Here's how the part is built. I have some questions about the finished solid (model axes, mm). A direction names the side the tool comes from. Coordinates: 2 decimals unless noted, no trailing zeros. Write each loop counter-clockwise with the first axis right and the second up, starting at its lowest first coordinate (ties: lowest second). Pieces come first, ordered by that corner, then holes.
```python
from build123d import *

# Parameters (mm, degrees)
F1_DEPTH = 87.5
F3_DEPTH = 100
F4_R     = 6.25
F5_DEPTH = 60.001
F6_R     = 3
F7_DEPTH = 120.001


with BuildPart() as f1:
    # F0 (on Top) → F1 (new body, symmetric)
    with BuildSketch(Plane.XY):
        with BuildLine():
            Line((20, 30), (-20, 30))
            ThreePointArc((-20, 30), (-27.071068, 27.071068), (-30, 20))
            Line((-30, 20), (-30, -20))
            ThreePointArc((-30, -20), (-27.071068, -27.071068), (-20, -30))
            Line((-20, -30), (20, -30))
            ThreePointArc((20, -30), (27.071068, -27.071068), (30, -20))
            Line((30, -20), (30, 20))
            ThreePointArc((30, 20), (27.071068, 27.071068), (20, 30))
        make_face()
        with BuildLine():
            ThreePointArc((-25, 20), (-23.535534, 23.535534), (-20, 25))
            Line((-20, 25), (20, 25))
            ThreePointArc((20, 25), (23.535534, 23.535534), (25, 20))
            Line((25, 20), (25, -20))
            ThreePointArc((25, -20), (23.535534, -23.535534), (20, -25))
            Line((20, -25), (-20, -25))
            ThreePointArc((-20, -25), (-23.535534, -23.535534), (-25, -20))
            Line((-25, -20), (-25, 20))
        make_face(mode=Mode.SUBTRACT)
    extrude(amount=F1_DEPTH, both=True)

    # F2 (on Front) → F3 (join, symmetric)
    with BuildSketch(Plane.XZ):
        with BuildLine():
            Line((-40, -27.5), (-80, -27.5))
            ThreePointArc((-80, -27.5), (-87.071068, -30.428932), (-90, -37.5))
            Line((-90, -37.5), (-90, -77.5))
            ThreePointArc((-90, -77.5), (-87.071068, -84.571068), (-80, -87.5))
            Line((-80, -87.5), (-40, -87.5))
            ThreePointArc((-40, -87.5), (-32.928932, -84.571068), (-30, -77.5))
            Line((-30, -77.5), (-30, -37.5))
            ThreePointArc((-30, -37.5), (-32.928932, -30.428932), (-40, -27.5))
        make_face()
        with BuildLine():
            ThreePointArc((-40, -32.5), (-36.464466, -33.964466), (-35, -37.5))
            Line((-35, -37.5), (-35, -77.5))
            ThreePointArc((-35, -77.5), (-36.464466, -81.035534), (-40, -82.5))
            Line((-40, -82.5), (-80, -82.5))
            ThreePointArc((-80, -82.5), (-83.535534, -81.035534), (-85, -77.5))
            Line((-85, -77.5), (-85, -37.5))
            ThreePointArc((-85, -37.5), (-83.535534, -33.964466), (-80, -32.5))
            Line((-80, -32.5), (-40, -32.5))
        make_face(mode=Mode.SUBTRACT)
    extrude(amount=F3_DEPTH, both=True)

    # F4 (on face) → F5 (cut, through all)
    with BuildSketch(Plane.YZ.offset(-30)):
        with Locations((-75, -57.5)):
            Circle(F4_R)
        with Locations((75, -57.5)):
            Circle(F4_R)
    extrude(amount=-F5_DEPTH, mode=Mode.SUBTRACT)

    # F6 (on face) → F7 (cut, through all)
    with BuildSketch(Plane.YZ.offset(30)):
        with Locations((0, 32.5)):
            Circle(F6_R)
        with Locations((0, 67.5)):
            Circle(F6_R)
    extrude(amount=-F7_DEPTH, mode=Mode.SUBTRACT)


solid = f1.part
```
1) Imagine slicing it at C-C on z = 32.5. Please give me the cut outline in (x, y).
Values follow:
outline: (-30, -20) arc R10 ccw to (-20, -30) - (20, -30) arc R10 ccw to (30, -20) - (30, -3) - (25, -3) - (25, -20) arc R5 cw to (20, -25) - (-20, -25) arc R5 cw to (-25, -20) - (-25, -3) - (-30, -3) - close; (-30, 3) - (-25, 3) - (-25, 20) arc R5 cw to (-20, 25) - (20, 25) arc R5 cw to (25, 20) - (25, 3) - (30, 3) - (30, 20) arc R10 ccw to (20, 30) - (-20, 30) arc R10 ccw to (-30, 20) - close
2) Imagine slicing it at B-B on z = -42. Please give me the cut outline in (x, y), then the cut area to 3 significant figures.
Values follow:
outline: (-90, -100) - (-85, -100) - (-85, 100) - (-90, 100) - close; (-35, -100) - (-30, -100) - (-30, -20) arc R10 ccw to (-20, -30) - (20, -30) arc R10 ccw to (30, -20) - (30, 20) arc R10 ccw to (20, 30) - (-20, 30) arc R10 ccw to (-30, 20) - (-30, 100) - (-35, 100) - close; hole (-25, -20) arc R5 ccw to (-20, -25) - (20, -25) arc R5 ccw to (25, -20) - (25, 20) arc R5 ccw to (20, 25) - (-20, 25) arc R5 ccw to (-25, 20) - close
area: 3,040 mm2
3) We'd pull the mould along Z, two halves only. Please class faces 1 (the face through (0, 25, 1)), 2 (the face through (-60, -1, -27.5)), 3 (the face through (-32.47, -69.04, -55.62)): pulls with the +Z half, pulls with the -Z half, needs draft (parallel to the pull), parting line crosses it, or undercut.
Values follow:
face 1: needs draft
face 2: pulls with the +Z half
face 3: undercut
4) On a 3-axis mill with a long thin cutter (end or side, diameter ignored), from which of +Z, -Z, +X, -X, +Y, -Y can I reach the whole of each face in a straight line? I mean faces 4 (the face through (-60, -1, -32.5)), 5 (the face through (0, 30, 1)), 6 (the face through (0, -25, 1)), 7 (the face through (0, -26, 87.5)), 8 (the face through (27.54, -2.21, 34.53)). Say none if no direction works.
Values follow:
face 4: +Y, -Y
face 5: +Z, -Z, +X, +Y
face 6: +Z, -Z
face 7: +Z, +X, -X, +Y, -Y
face 8: +X, -X
5) Will these pins go through, and if not, where does the flat tip stop? pin 1 (20 mm diameter, centred on y = 73, z = -54.5, fed in from +X); pin 2 (10 mm diameter, centred on y = 75, z = -57.5, fed in from +X); pin 3 (12 mm diameter, centred on x = -60.5, y = 18, fed in from +Z); pin 4 (3 mm diameter, centred on x = 12.5, z = -39, fed in from -Y).
Values follow:
pin 1: stops at x = -30
pin 2: passes through
pin 3: stops at z = -27.5
pin 4: stops at y = -30
6) I need wall thicknesses on probe 1 along Z at (x, y) = (-27.5, 0); probe 2 along Y at (x, z) = (-11.5, -12.5). Which ranges of each line are inside material? Lowest first, please.
Values follow:
probe 1: z = -87.5 to 29.5, 35.5 to 64.5, 70.5 to 87.5
probe 2: y = -30 to -25, 25 to 30
7) Imagine slicing it at A-A on y = -14.5. Please give me the cut outline in (x, z), then the cut area to 3 significant figures.
Values follow:
outline: (-90, -77.5) arc R10 ccw to (-80, -87.5) - (-40, -87.5) arc R10 ccw to (-30, -77.5) - (-30, -87.5) - (-25, -87.5) - (-25, 87.5) - (-30, 87.5) - (-30, -37.5) arc R10 ccw to (-40, -27.5) - (-80, -27.5) arc R10 ccw to (-90, -37.5) - close; (25, -87.5) - (30, -87.5) - (30, 87.5) - (25, 87.5) - close; hole (-85, -77.5) arc R5 ccw to (-80, -82.5) - (-40, -82.5) arc R5 ccw to (-35, -77.5) - (-35, -37.5) arc R5 ccw to (-40, -32.5) - (-80, -32.5) arc R5 ccw to (-85, -37.5) - close
area: 2,790 mm2
8) Imagine slicing it at D-D on x = -64. Please give me the cut outline in (y, z), then the cut area to 3 significant figures.
Values follow:
outline: (-100, -87.5) - (100, -87.5) - (100, -82.5) - (-100, -82.5) - close; (-100, -32.5) - (100, -32.5) - (100, -27.5) - (-100, -27.5) - close
area: 2,000 mm2
